For this review, take the finished solid that the model builds, in its own axes (mm). Coordinates: 2 decimals unless noted, no trailing zeros. Order: outer loops, then holes, each group sorted by start corner. A loop starts at its lowest first (then second) coordinate and runs counter-clockwise, first axis right, second up. Notation, with made-up numbers: (26.25, 51.5) - (51.25, 51.5) arc R14 cw to (51.25, 73.5) - close; hole circle Ø11 at (70, -15). An arc over 180 degrees is marked (long way). One line per item, written item: value. Start each with the question number.
(1) Consider section C-C on x = 0.45. Count the separate pieces of the cut face and the enclosed holes in it, then the cut area to 3 significant figures.
(2) Consider section D-D on y = 52. Write out the cut boundary in (x, z).
(3) Consider section A-A on z = -12.7. Write out the cut boundary in (x, y).
(4) To check wall thickness, follow line 1 along Z through (x, y) = (0.3, 0); line 2 along Y through (x, z) = (0.75, -69); line 3 along Y through (x, z) = (1.2, -209.55). State the ranges of each line that lie inside material, in increasing order.
(5) Clearance check with a flat-ended pin moving along its axis: pin 1 (0.5 mm diameter, centred on x = 1, z = -35.5, fed in from +Y). State where the tip first meets the part, or that it passes through.
(6) Consider section B-B on y = 0. Write out the cut boundary in (x, z).
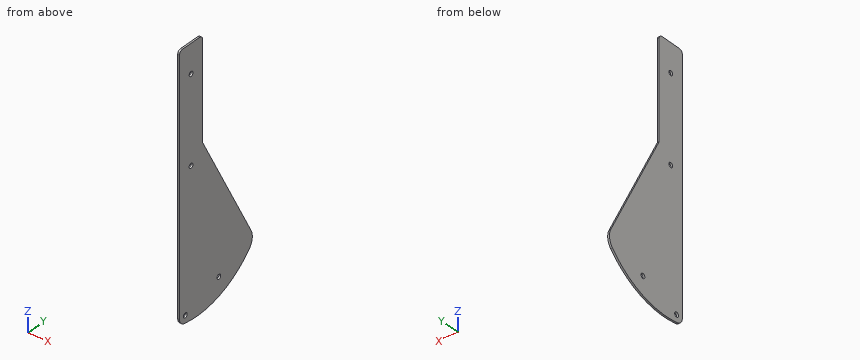
Autodesk Inventor part; units mm, degrees
ref_plane "YZ Plane" through (0, 0, 0) normal (1, 0, 0) x (0, 1, 0)
ref_plane "XZ Plane" through (0, 0, 0) normal (0, 1, 0) x (-1, 0, 0)
ref_plane "XY Plane" through (0, 0, 0) normal (0, 0, 1) x (1, 0, 0)
sketch "main" plane through (0, 0, 0) normal (0, 0, 1) x (1, 0, 0)
  circle A0 centre (-31.9195, -99.4713) radius 2.0955
  arc A1 (-38.2695, -99.4713) -> (-33.0376, -105.722) centre (-31.9195, -99.4713) ccw
  arc A2 (-33.0376, -105.722) -> (38.5686, -81.1636) centre (-19.3218, -29.0418) ccw
  line L0 (40.3562, -66.7269) -> (-12.8695, 33.8787)
  line L1 (-12.8695, 33.8787) -> (-12.8695, 119.6037)
  line L2 (-16.0445, 122.7787) -> (-35.0945, 122.7787)
  line L3 (-38.2695, 119.6037) -> (-38.2695, -99.4713)
  arc A3 (38.5686, -81.1636) -> (40.3562, -66.7269) centre (29.1304, -72.6659) ccw
  circle A4 centre (-25.5695, 21.1787) radius 2.0955
  arc A5 (-12.8695, 119.6037) -> (-16.0445, 122.7787) centre (-16.0445, 119.6037) ccw
  circle A6 centre (5.0055, -86.7713) radius 2.0955
  circle A7 centre (-25.5695, 97.3787) radius 2.0955
  arc A8 (-35.0945, 122.7787) -> (-38.2695, 119.6037) centre (-35.0945, 119.6037) ccw
  point P0 (-9.1863, -18.3686)
  point P1 (44.2418, -74.0713)
  dimension "d0" = 4.191
  dimension "d1" = 12.7
  dimension "d3" = 4.191
  dimension "d4" = 3.175
  dimension "d5" = 4.191
  dimension "d17" = 4.191
  dimension "d18" = 3.175
sketch "Sketch1" plane through (0, 0, 0) normal (1, 0, 0) x (0, 1, 0)
  circle A0 centre (-6.35, -209.55) radius 2.0955
  arc A1 (-12.7, -209.55) -> (-7.4681, -215.8008) centre (-6.35, -209.55) ccw
  arc A2 (-7.4681, -215.8008) -> (64.1381, -191.2423) centre (6.2477, -139.1205) ccw
  line L0 (65.9257, -176.8056) -> (12.7, -76.2)
  line L1 (12.7, -76.2) -> (12.7, 9.525)
  line L2 (9.525, 12.7) -> (-9.525, 12.7)
  line L3 (-12.7, 9.525) -> (-12.7, -209.55)
  arc A3 (64.1381, -191.2423) -> (65.9257, -176.8056) centre (54.7, -182.7446) ccw
  circle A4 centre (0, -88.9) radius 2.0955
  arc A5 (12.7, 9.525) -> (9.525, 12.7) centre (9.525, 9.525) ccw
  circle A6 centre (30.575, -196.85) radius 2.0955
  circle A7 centre (0, -12.7) radius 2.0955
  arc A8 (-9.525, 12.7) -> (-12.7, 9.525) centre (-9.525, 9.525) ccw
  point P0 (0, 0)
extrude "Extrusion1" add sketch "Sketch1" along normal blind 1.5875
equation "\"BendRadius\" = Thickness"
equation "\"BendReliefWidth\" = Thickness"
equation "\"BendReliefDepth\" = 0.5 * Thickness"
equation "\"CornerReliefSize\" = 4 * Thickness"
equation "\"MinimumRemnant\" = 2 * Thickness"
equation "\"TransitionRadius\" = BendRadius"
equation "\"JacobiRadiusSize\" = BendRadius"
equation "\"GapSize\" = Thickness"
properties part number "gusset_no_motor" material "Acetal Resin, White"
Geometry check:
1. separate pieces: 1
1. enclosed holes: 4
1. area: 10,100 mm^2
2. outline: (0, -202.17) - (1.59, -202.17) - (1.59, -150.48) - (0, -150.48) - close
3. outline: (0, -12.7) - (1.59, -12.7) - (1.59, -2.1) - (0, -2.1) - close; (0, 2.1) - (1.59, 2.1) - (1.59, 12.7) - (0, 12.7) - close
4. line 1: z = -216.77 to -91, -86.8 to -14.8, -10.6 to 12.7
4. line 2: y = -12.7 to 12.7
4. line 3: y = -12.7 to -8.45, -4.25 to 39.53
5. pin 1: stops at y = 12.7
6. outline: (0, -216.77) - (1.59, -216.77) - (1.59, -91) - (0, -91) - close; (0, -86.8) - (1.59, -86.8) - (1.59, -14.8) - (0, -14.8) - close; (0, -10.6) - (1.59, -10.6) - (1.59, 12.7) - (0, 12.7) - close
